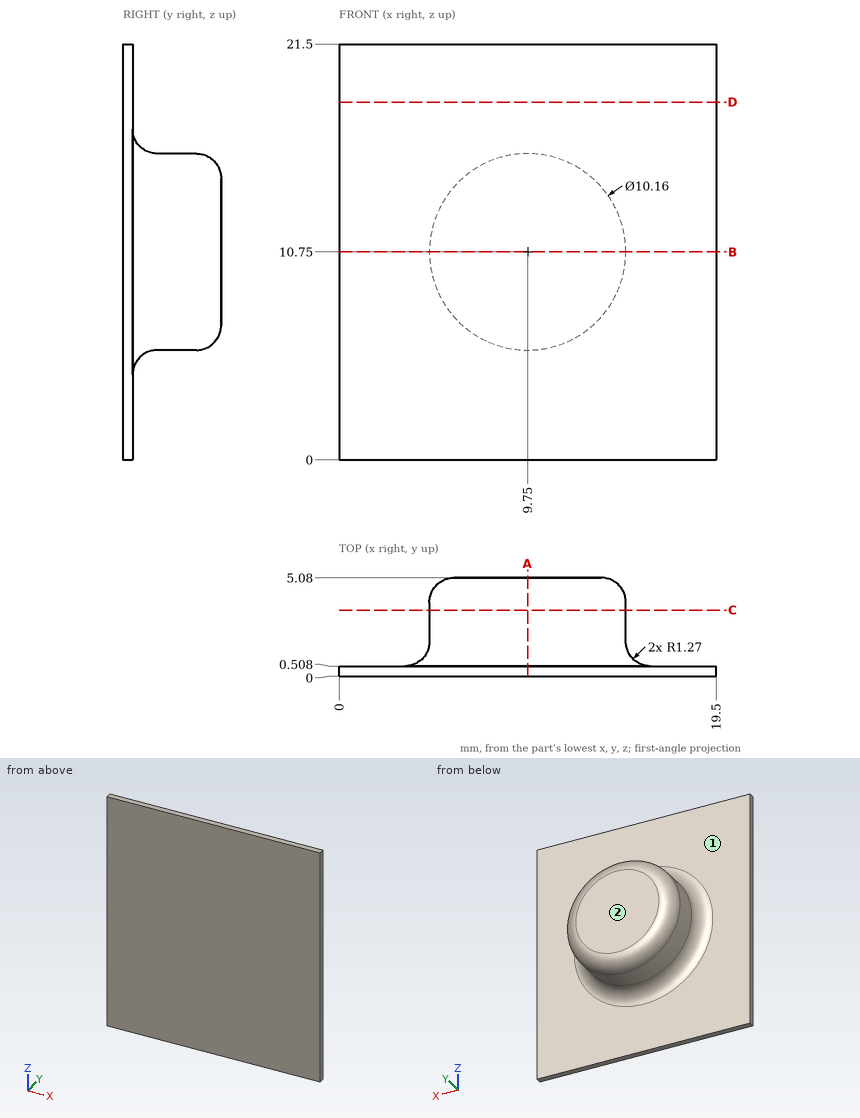
Study the drawing (mm; zero at the part's minimum x, y, z) and answer. A direction names the side the tool comes from. Round coordinates to 2 decimals unless told otherwise and drop trailing zeros. Order: outer loops, then holes, each group sorted by start corner. A loop starts at its lowest first (then second) coordinate and runs counter-clockwise, first axis right, second up. Notation, with made-up numbers: (89, 34.25) - (98, 34.25) arc R38 ccw to (98, 72.25) - close; hole circle Ø2 at (17.25, -4). An arc over 180 degrees is marked (long way). Use one line per item in the form item = value. Start each with the question number.
(1) A flat-ended cylindrical pin translates along its axis: pin 1 Ø1 at (x, z) = (16.5, 5) entering from +Y. Find the tip coordinate at first contact, or state that the pin passes through.
(2) The part is cut by section C-C (y = 3.4). Give the vertices of the cut face in (x, z), then the cut area to 3 significant figures.
(3) For the marked faces 1 and 2, determine the directions among +Z, -Z, +X, -X, +Y, -Y from which every point of the face is accessible in a straight line to the end or side of a thin tool.
(4) The part is cut by section A-A (x = 9.75). Give the vertices of the cut face in (y, z), then the cut area to 3 significant figures.
(5) The part is cut by section D-D (z = 18.5). Give the vertices of the cut face in (x, y), then the cut area to 3 significant figures.
(6) The part is cut by section B-B (z = 10.75). Give the vertices of the cut face in (x, y), then the cut area to 3 significant figures.
(7) Find the intervals of material crossed by line 1 along Y through (x, z) = (17.5, 7.25); line 2 along Z through (x, y) = (12.75, 4); line 3 along X through (y, z) = (2.35, 10), in increasing order. Write a range as from..to.
Checked values:
q1.pin_1 = 0.51
q2.outline = circle Ø10.16 at (9.75, 10.75)
q2.area = 81.1 mm^2
q3.face_1 = +Y
q3.face_2 = +Z, -Z, +X, -X, +Y
q4.outline = (0, 0) - (0.51, 0) - (0.51, 4.4) arc R1.27 cw to (1.78, 5.67) - (3.81, 5.67) arc R1.27 ccw to (5.08, 6.94) - (5.08, 14.56) arc R1.27 ccw to (3.81, 15.83) - (1.78, 15.83) arc R1.27 cw to (0.51, 17.1) - (0.51, 21.5) - (0, 21.5) - close
q4.area = 57.4 mm^2
q5.outline = (0, 0) - (19.5, 0) - (19.5, 0.51) - (0, 0.51) - close
q5.area = 9.91 mm^2
q6.outline = (0, 0) - (19.5, 0) - (19.5, 0.51) - (16.1, 0.51) arc R1.27 cw to (14.83, 1.78) - (14.83, 3.81) arc R1.27 ccw to (13.56, 5.08) - (5.94, 5.08) arc R1.27 ccw to (4.67, 3.81) - (4.67, 1.78) arc R1.27 cw to (3.4, 0.51) - (0, 0.51) - close
q6.area = 56.4 mm^2
q7.line_1 = 0..0.51
q7.line_2 = 6.67..14.83
q7.line_3 = 4.73..14.77
